from build123d import *

# Parameters (mm, degrees)
SKETCH1_W           = 277
SKETCH1_H           = 300
BOSS_EXTRUDE1_DEPTH = 6
BOSS_EXTRUDE2_DEPTH = 7
BOSS_EXTRUDE3_DEPTH = 5
CUT_EXTRUDE1_DEPTH  = 19


with BuildPart() as part:
    # Sketch1 → Boss-Extrude1 (new body)
    with BuildSketch(Plane.XY):
        Rectangle(SKETCH1_W, SKETCH1_H)
    extrude(amount=BOSS_EXTRUDE1_DEPTH)

    # Sketch3 → Boss-Extrude2 (add)
    with BuildSketch(Plane(origin=(0, 0, 0), x_dir=(-1, 0, 0), z_dir=(0, 0, -1))):
        Polygon((-103.5, -130), (-34.217967697, -140), (-32.789396269, -130.102566814), (-102.071428571, -120.102566814), align=None)
    boss_extrude2 = extrude(amount=BOSS_EXTRUDE2_DEPTH)

    # Sketch4 → Boss-Extrude3 (add)
    with BuildSketch(Plane(origin=(0, 0, -7), x_dir=(-1, 0, 0), z_dir=(0, 0, -1))):
        Polygon((-102.071428571, -120.102566814), (-32.789396269, -130.102566814), (-34.932253412, -144.948716593), (-104.214285714, -134.948716593), align=None)
    boss_extrude3 = extrude(amount=BOSS_EXTRUDE3_DEPTH)

    # Sketch2 → Cut-Extrude1 (cut, through all)
    with BuildSketch(Plane.XY.offset(6)):
        with BuildLine():
            Line((133.5, 123), (133.5, 88))
            ThreePointArc((133.5, 88), (148.5, 73), (163.5, 88))
            Line((163.5, 88), (163.5, 123))
            ThreePointArc((163.5, 123), (148.5, 138), (133.5, 123))
        make_face()
    cut_extrude1 = extrude(amount=-CUT_EXTRUDE1_DEPTH, mode=Mode.SUBTRACT)

    # Mirror1: Boss-Extrude2, Boss-Extrude3, Cut-Extrude1 across plane
    add(boss_extrude2.mirror(Plane(origin=(0, 0, 0), x_dir=(0, 0, 1), z_dir=(1, 0, 0))))
    add(boss_extrude3.mirror(Plane(origin=(0, 0, 0), x_dir=(0, 0, 1), z_dir=(1, 0, 0))))
    add(cut_extrude1.mirror(Plane(origin=(0, 0, 0), x_dir=(0, 0, 1), z_dir=(1, 0, 0))), mode=Mode.SUBTRACT)


solid = part.part
Check sheet for the modelled part. Datum: model origin and axes. Units: mm. A direction names the side the tool comes from. Give positions to 0.01 mm unless a question says otherwise; leave off trailing zeros. Order: outer loops, then holes, each group sorted by start corner. A loop starts at its lowest first (then second) coordinate and runs counter-clockwise, first axis right, second up. Notation, with made-up numbers: M 81.5,-18 L 93.5,-18 A33 cw 93.5,12 Z; hole C 39.5,62.25 d3. An arc over 180 degrees is marked long. Answer as CSV lines item,"result". Start each with the question number.
Item 1: Cross-section at D-D on x = 52.5. Enter the section's corners in (y, z), plus the area to 3 significant figures.
Item 2: Mould release check, pull along X, two halves, no side actions. Record for faces 1 (the face through (67.92, -125.03, -5.92)), 2 (the face through (68, -132, -12)), 3 (the face through (-69.34, -134.93, -3.45)): +X half, -X half, draft (parallel to the pull), parting line (faces both ways), or undercut.
Item 3: Gauge pin test, flat ends, axial feed: P1, Ø5, axis at x = -43, z = -6, coming from the -Y side; P2, Ø2, axis at x = -49, z = -3, coming from the +Y side; P3, Ø8, axis at y = 99, z = -1.5, coming from the -X side. Record the tip position at first contact, or that the pin passes through.
Item 4: Cross-section at A-A on z = -2.75. Enter the section's corners in (x, y), plus the area to 3 significant figures.
Item 5: Cross-section at B-B on x = -24.5. Enter the section's corners in (y, z).
Item 6: Cross-section at C-C on y = -1.5. Enter the section's corners in (x, z).
Item 7: Tool access check on faces 4 (the face through (-69.09, -140.02, -9.46)), 5 (the face through (-67.92, -125.03, -5.92)), 6 (the face through (69, -138, -7)). Record the directions out of +Z, -Z, +X, -X, +Y, -Y that give a thin tool (end or side, any length) a straight path to the whole face; none if there is none.
Item 8: Thickness scan on line 1 (Z direction, x = 54, y = 84); line 2 (Y direction, x = -38.5, z = -10.5); line 3 (Y direction, x = 90.5, z = -4). Record the ranges inside material, lowest first. Write a range as [from, to].
Established:
1,outline,"M -150,0 L -137.36,0 L -137.36,-7 L -142.41,-7 L -142.41,-12 L -127.26,-12 L -127.26,0 L 150,0 L 150,6 L -150,6 Z"
1,area,"1,950 mm^2"
2,face 1,"undercut"
2,face 2,"draft"
2,face 3,"-X half"
3,P1,"stops at y = -144.11"
3,P2,"stops at y = -127.62"
3,P3,"stops at x = -133.5"
4,outline,"M -103.5,-130 L -34.22,-140 L -32.79,-130.1 L -102.07,-120.1 Z; M 32.79,-130.1 L 34.22,-140 L 103.5,-130 L 102.07,-120.1 Z"
4,area,"1,400 mm^2"
5,outline,"M -150,0 L 150,0 L 150,6 L -150,6 Z"
6,outline,"M -138.5,0 L 138.5,0 L 138.5,6 L -138.5,6 Z"
7,face 4,"-Z, -X, -Y"
7,face 5,"-Z, +Y"
7,face 6,"+X, -Y"
8,line 1,"z = [0, 6]"
8,line 2,"y = [-144.43, -129.28]"
8,line 3,"y = [-131.88, -121.77]"
